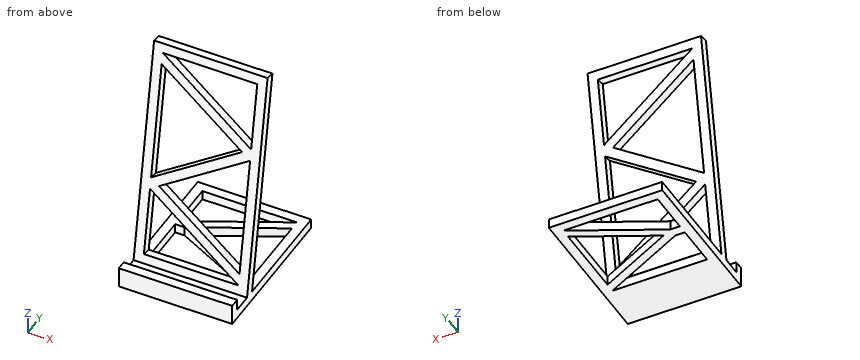
```python
from build123d import *

# Parameters (mm, degrees)
F1_DEPTH = 38.1
F3_DEPTH = 25.4
F5_DEPTH = 6.35


with BuildPart() as f1:
    # F0 (on Right) → F1 (new body, symmetric)
    with BuildSketch(Plane.YZ):
        Polygon((-38.0986895752, 13.97), (-44.4486895752, 13.97), (-44.4486895752, 0), (57.2492694102, 0), (57.2492694102, 6.35), (-18.9507305898, 6.35), (7.3188219328, 155.3320356309), (1.0652927012, 156.4347015591), (-25.3986895752, 6.35), (-38.0986895752, 6.35), align=None)
    extrude(amount=F1_DEPTH, both=True)

    # F2 (on face) → F3 (cut)
    with BuildSketch(Plane.XY.offset(6.35)):
        Polygon((-31.75, -12.6007305898), (31.75, -12.6007305898), (-25.4, 15.9742694102), (-31.75, 15.9742694102), align=None)
        Polygon((31.75, -6.2507305898), (31.75, 44.5492694102), (-19.05, 19.1492694102), align=None)
        Polygon((-25.4, 22.3242694102), (31.75, 50.8992694102), (-31.75, 50.8992694102), (-31.75, 22.3242694102), align=None)
    extrude(amount=-F3_DEPTH, mode=Mode.SUBTRACT)

    # F4 (on face) → F5 (cut, through all)
    with BuildSketch(Plane(origin=(0, -25.7187393284, 4.5349076534), x_dir=(1, 0, 0), z_dir=(0, -0.984807753, 0.1736481777))):
        Polygon((31.75, 147.8930930718), (-31.75, 147.8930930718), (31.75, 102.4655281848), align=None)
        Polygon((26.0160516338, 98.7599313647), (-31.75, 140.0854598506), (-31.75, 61.4282911798), align=None)
        Polygon((31.75, 16.0007262929), (31.75, 94.6578949637), (-26.0160516338, 57.3262547788), align=None)
        Polygon((31.75, 8.1930930718), (-31.75, 53.6206579587), (-31.75, 8.1930930718), align=None)
    extrude(amount=-F5_DEPTH, mode=Mode.SUBTRACT)


solid = f1.part
```
Model file for the job. Use its own axes, mm. Round coordinates to 2 decimals unless told otherwise and drop trailing zeros. Write each loop counter-clockwise with the first axis right and the second up, starting at its lowest first coordinate (ties: lowest second). Pieces come first, ordered by that corner, then holes. Notation, with made-up numbers: (7, 55) - (60, 55) arc R24 ccw to (60, 73) - close; hole circle Ø4 at (70, 68.5). An arc over 180 degrees is marked (long way). One line per item, written item: value.
(1) Cut at D-D, the plane y = 48. Give the cut face in (x, z), plus the area to 3 significant figures.
Values follow:
outline: (-38.1, 0) - (-31.75, 0) - (-31.75, 6.35) - (-38.1, 6.35) - close; (25.95, 0) - (38.1, 0) - (38.1, 6.35) - (25.95, 6.35) - close
area: 117 mm²
(2) Drop flat-ended pins along their axis: P1, Ø2, axis at x = -3.5, z = 129, coming from the -Y side; P2, Ø2.5, axis at x = 16, z = 10.5, coming from the +Y side; P3, Ø14, axis at x = 19, y = -30.5, coming from the +Z side; P4, Ø10, axis at y = 7.5, z = 99.5, coming from the +X side. Give the stop position or say it passes through.
Values follow:
P1: stops at y = -3.95
P2: stops at y = -18.04
P3: stops at z = 12.6
P4: passes through
(3) Cut at C-C, the plane x = -22. Give the number of separate pieces and of enclosed holes in the cut face, plus the area to 3 significant figures.
Values follow:
separate pieces: 7
enclosed holes: 0
area: 579 mm²
(4) Cut at B-B, the plane y = 3. Give the cut face in (x, z).
Values follow:
outline: (-38.1, 0) - (-31.75, 0) - (-31.75, 6.35) - (-38.1, 6.35) - close; (-38.1, 130.84) - (-31.75, 130.84) - (-31.75, 141.72) - (-16.77, 130.84) - (-5.86, 130.84) - (-31.75, 149.65) - (31.75, 149.65) - (31.75, 130.84) - (38.1, 130.84) - (38.1, 156.09) - (-38.1, 156.09) - close; (0.55, 0) - (13.25, 0) - (13.25, 6.35) - (0.55, 6.35) - close; (31.75, 0) - (38.1, 0) - (38.1, 6.35) - (31.75, 6.35) - close
(5) Wall check: probe 1 along Y at (x, z) = (8.5, 7); probe 2 along Z at (x, y) = (-0.5, -35.5); probe 3 along Z at (x, y) = (21, 1.5). Give the ranges that are in metal, low to high.
Values follow:
probe 1: y = -44.45 to -38.1, -25.28 to -18.84
probe 2: z = 0 to 6.35
probe 3: z = 149.91 to 156.36
(6) Cut at A-A, the plane z = 91.5. Give the cut face in (x, y).
Values follow:
outline: (-38.1, -10.38) - (-31.75, -10.38) - (-31.75, -3.94) - (-38.1, -3.94) - close; (9.84, -10.38) - (21.92, -10.38) - (23.65, -3.94) - (11.57, -3.94) - close; (31.75, -10.38) - (38.1, -10.38) - (38.1, -3.94) - (31.75, -3.94) - close
